Autodesk Fusion 360 part; units mm, degrees
sketch "Sketch1" plane through (0, 0, 0) normal (0, 1, 0) x (1, 0, 0)
  circle A0 centre (0, 0) radius 32.5
  circle A1 centre (0, 0) radius 28.5
  dimension "d1" = 65
  dimension "d2" = 57
extrude "Extrude1" add sketch "Sketch1" along normal blind 10 makes body 1
sketch "Sketch2" plane through (0, 10, 0) normal (0, 1, 0) x (-1, 0, 0)
  circle A0 centre (0, 0) radius 28.5
  circle A1 centre (0, 0) radius 32.5
  circle A2 centre (0, 0) radius 28.5
  circle A3 centre (0, 0) radius 28
  circle A4 centre (0, 0) radius 27
  dimension "d5" = -0.5
  dimension "d8" = -1.5
extrude "Extrude3" add sketch "Sketch2" along normal blind 30 and the other way blind 5 separate body contours A3 makes body 2
sketch "Sketch3" plane through (0, 0, 0) normal (0, -1, 0) x (1, 0, 0)
  circle A0 centre (0, 0) radius 28.5
  circle A1 centre (0, 0) radius 32.5
  circle A2 centre (0, 0) radius 28.5
  circle A3 centre (0, 0) radius 28
extrude "Extrude4" add sketch "Sketch3" against normal blind 10 contours A0 A2 bodies 1 2
fillet "Fillet1" radius 1 1 edges at (26.1052, 5, 10.1252) on bodies 1
chamfer "Chamfer1" distance 0.5 angle 45 1 edges at (26.1052, 40, -10.1252) on bodies 1 2
equation "d8 = -0.5 mm - 1 mm"
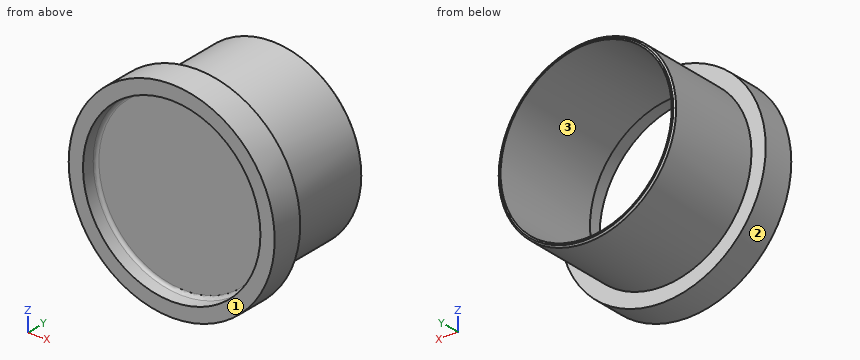
Source: CAD feature listing. Evaluate the final solid. Frame: model axes, mm. Face numbers are marked on the shaded views. Give positions to 0.01 mm unless a question says otherwise; leave off trailing zeros. Loops run counter-clockwise (first coordinate to the right, second up) from the corner with the lowest first, then second, coordinate; pieces in that order, holes last. Notation, with made-up numbers: (9.5, 31) -> (22.5, 31) arc R25 cw to (22.5, 47) -> close; hole circle Ø2 at (44.5, 78). An arc over 180 degrees is marked (long way). Use a Markdown table: item, result. Add a question column.
1) Line query: line 1 along Z through (x, y) = (0, 2.3); line 2 along Z through (x, y) = (0, 21); line 3 along X through (y, z) = (14.5, 22.5). Output: solid intervals per line, ascending. Write a range as [from, to].
2) Pull-direction query (Z, two-part tool) for the marked faces 1, 2 and 3; classes: +Z half, -Z half, draft (parallel to the pull), parting line (faces both ways), or undercut.
3) Section query C-C, the plane y = 32. Return the cut outline in (x, z).
4) First-contact query: pin 1 (10 mm diameter, centred on y = 23, z = 3, fed in from -X); pin 2 (1 mm diameter, centred on y = 24.5, z = -10.5, fed in from +X); pin 3 (12 mm diameter, centred on y = 32.5, z = -8, fed in from -X). Flat tips, straight axial feed; report the tip coordinate or a pass-through.
Numbers:
| question | item | result |
|---|---|---|
| 1 | line 1 | z = [-32.5, -28], [28, 32.5] |
| 1 | line 2 | z = [-28, -27], [27, 28] |
| 1 | line 3 | x = [-16.67, -14.92], [14.92, 16.67] |
| 2 | face 1 | draft |
| 2 | face 2 | parting line |
| 2 | face 3 | undercut |
| 3 | outline | circle Ø56 at (0, 0); hole circle Ø54 at (0, 0) |
| 4 | pin 1 | stops at x = -28 |
| 4 | pin 2 | stops at x = 26.15 |
| 4 | pin 3 | stops at x = -27.93 |
